Input: dimensioned drawing with shaded views. Units: mm. Origin: part minimum x, y, z. A direction names the side the tool comes from. Give positions to 0.01 mm unless a question says otherwise; leave off trailing zeros. Write each loop counter-clockwise with the first axis right and the second up, starting at its lowest first coordinate (ties: lowest second). Pieces come first, ordered by that corner, then holes.
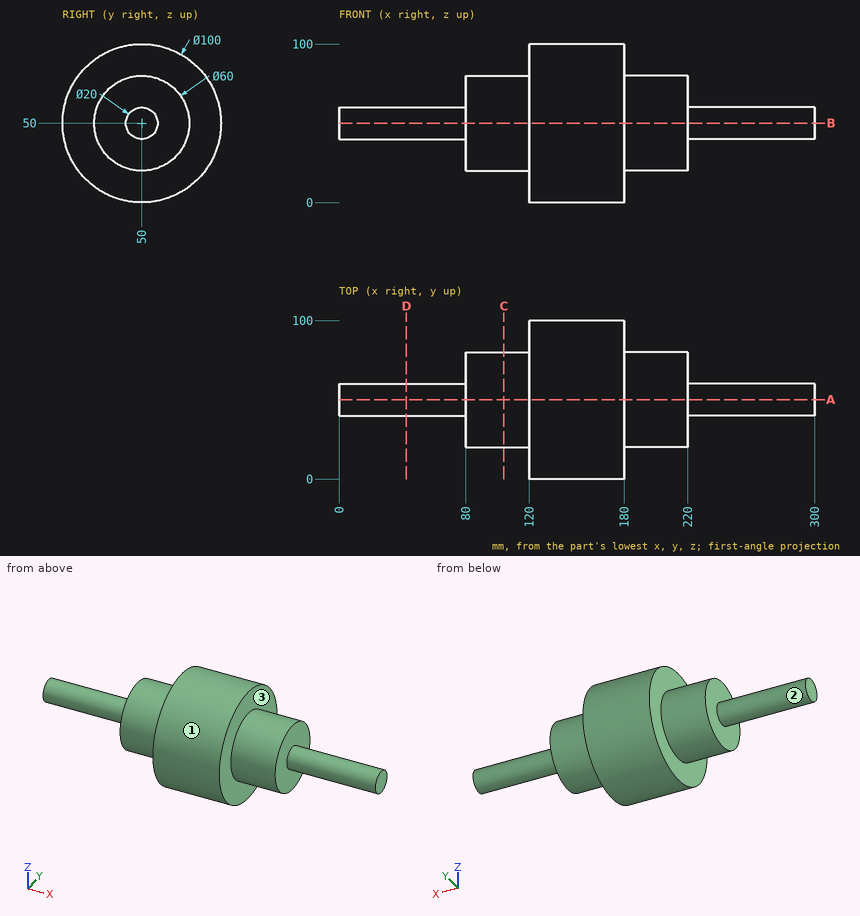
1. Cut plane A-A, the plane y = 50. Return the cut outline in (x, z).
2. Access query for the marked faces 1, 2 and 3. Directions: +Z, -Z, +X, -X, +Y, -Y. A direction counts if a zero-diameter tool reaches every point of the face in a straight line with its end or side. Return the directions, or none.
3. Cut plane D-D, the plane x = 42.5. Return the cut outline in (y, z).
4. Cut plane C-C, the plane x = 104. Return the cut outline in (y, z).
5. Line query: L1, parallel to X at y = 27.5, z = 94; L2, parallel to X at y = 45, z = 25; L3, parallel to Z at x = 162.5, y = 4. Output: solid intervals per line, ascending.
6. Contact query for flat-ended pins moving along their axis: P1, Ø2, axis at y = 68.5, z = 83, coming from the +X side; P2, Ø12, axis at y = 72.5, z = 30, coming from the +X side; P3, Ø5, axis at x = 85.5, z = 47, coming from the +Y side. Output: stop coordinate, or through.
Response values:
1. outline: (0, 40) - (80, 40) - (80, 20) - (120, 20) - (120, 0) - (180, 0) - (180, 20) - (220, 20) - (220, 40) - (300, 40) - (300, 60) - (220, 60) - (220, 80) - (180, 80) - (180, 100) - (120, 100) - (120, 80) - (80, 80) - (80, 60) - (0, 60) - close
2. face 1: +X, -X
2. face 2: -X
2. face 3: +X
3. outline: circle Ø20 at (50, 50)
4. outline: circle Ø60 at (50, 50)
5. L1: x = 120 to 180
5. L2: x = 80 to 220
5. L3: z = 30.4 to 69.6
6. P1: stops at x = 180
6. P2: stops at x = 220
6. P3: stops at y = 80
